from build123d import *

# Parameters (mm, degrees)
F1_DEPTH = 20
F0_W     = 75
F0_H     = 20
F2_DEPTH = 15
F4_DEPTH = 10
F6_DEPTH = 5
F7_D     = 6.3
F7_DEPTH = 15
F7_TIP   = 1.8927109499


with BuildPart() as f1:
    # F0 (on Front) → F1 (new body)
    with BuildSketch(Plane.XZ):
        Polygon((-25, 35), (-45, 35), (-45, -40), (-25, -40), (-25, -10), (-25, 10), align=None)
    extrude(amount=F1_DEPTH)

    # F0 (on Front) → F2 (join)
    with BuildSketch(Plane.XZ):
        with Locations((12.5, 0)):
            Rectangle(F0_W, F0_H)
    extrude(amount=F2_DEPTH)

    # F3 (on Top) → F4 (join, symmetric)
    with BuildSketch(Plane.XY):
        with BuildLine():
            Line((-25, -15), (-25, -20))
            ThreePointArc((-25, -20), (1.7392618935, -34.8926189355), (25, -15))
            Line((25, -15), (0, -15))
            Line((0, -15), (-25, -15))
        make_face()
    extrude(amount=F4_DEPTH, both=True)

    # F5 (on face) → F6 (cut)
    with BuildSketch(Plane.XY.offset(10)):
        Polygon((5.2573132542, -21.9703298494), (0.009059209, -18.9362188631), (-5.2426850057, -21.9642846986), (-5.2461751751, -28.0264615203), (0.0020788701, -31.0605725067), (5.2538230847, -28.0325066712), align=None)
    extrude(amount=-F6_DEPTH, mode=Mode.SUBTRACT)

    # F7
    with Locations(Plane.XY.offset(10)):
        with Locations((0.0055690395, -24.9983956849)):
            Hole(F7_D / 2, depth=F7_DEPTH)
            with Locations((0, 0, -(F7_DEPTH + F7_TIP / 2))):  # 118° drill point
                Cone(0, F7_D / 2, F7_TIP, mode=Mode.SUBTRACT)


with BuildPart() as f8_1:
    # F8: instance of F1
    add(f1.part.mirror(Plane(origin=(50, -7.5, 0), x_dir=(0, 1, 0), z_dir=(1, 0, 0))))


solid = f8_1.part
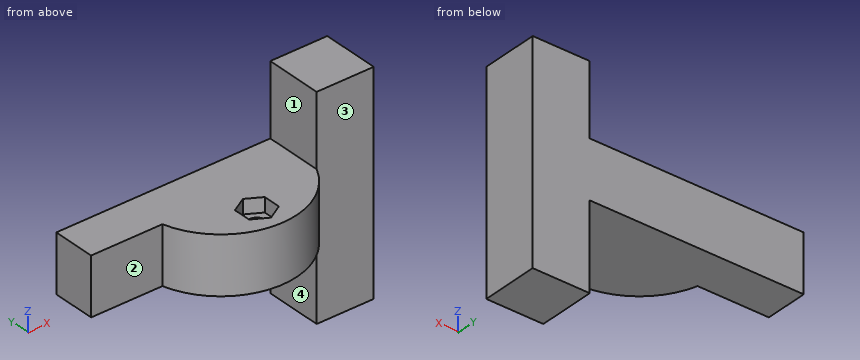
The model under review builds one solid part; all positions refer to its coordinate system, in mm. Face numbers are marked on the shaded views. A direction names the side the tool comes from. Round coordinates to 2 decimals unless told otherwise and drop trailing zeros. Write each loop counter-clockwise with the first axis right and the second up, starting at its lowest first coordinate (ties: lowest second). Pieces come first, ordered by that corner, then holes. Notation, with made-up numbers: M -2,-34.75 L 41,-34.75 A27 cw 41,-9.75 Z; hole C -3.5,78 d9. An arc over 180 degrees is marked long. Use a Markdown table: item, result. Add a question column.
Q1. We need section A-A, the plane y = -7.5. State the section outline as (x, z) points.
Q2. To check wall thickness, follow line 1 (X direction, y = -5, z = 22); line 2 (Z direction, x = 111, y = -26); line 3 (Y direction, x = 72, z = -4.5). State the ranges of each line that lie inside material, in increasing order.
Q3. We need section B-B, the plane z = 16.5. State the section outline as (x, y) points.
Q4. We need section C-C, the plane x = 134. State the section outline as (y, z) points, plus the area to 3 significant figures.
Q5. Insertion check: pin 1 (10.5 mm diameter, centred on x = 69.5, y = -11.5, fed in from -Z); pin 2 (6 mm diameter, centred on y = -7, z = 21, fed in from -X); pin 3 (2 mm diameter, centred on y = -24, z = -7, fed in from +X). Each pin has a flat end and moves straight along its axis. Give the tip position at first contact, or say it passes through.
Q6. Machinability: for the marked faces 1, 2, 3 and 4, which of the approach directions +Z, -Z, +X, -X, +Y, -Y give a long, thin tool a straight path to every point of the face, cutting with its end or side? Answer none if there is none.
Findings below:
| question | item | result |
|---|---|---|
| 1 | outline | M 50,-10 L 125,-10 L 125,-40 L 145,-40 L 145,35 L 125,35 L 125,10 L 50,10 Z |
| 2 | line 1 | x = 125 to 145 |
| 2 | line 2 | z = -10 to 10 |
| 2 | line 3 | y = -15 to 0 |
| 3 | outline | M 125,-20 L 145,-20 L 145,0 L 125,0 Z |
| 4 | outline | M -20,-40 L 0,-40 L 0,35 L -20,35 Z |
| 4 | area | 1,500 mm² |
| 5 | pin 1 | stops at z = -10 |
| 5 | pin 2 | stops at x = 125 |
| 5 | pin 3 | stops at x = 123.29 |
| 6 | face 1 | +Z, -X, +Y, -Y |
| 6 | face 2 | +Z, -Z, -X, -Y |
| 6 | face 3 | +Z, -Z, +X, -Y |
| 6 | face 4 | -Z, -X, +Y, -Y |
